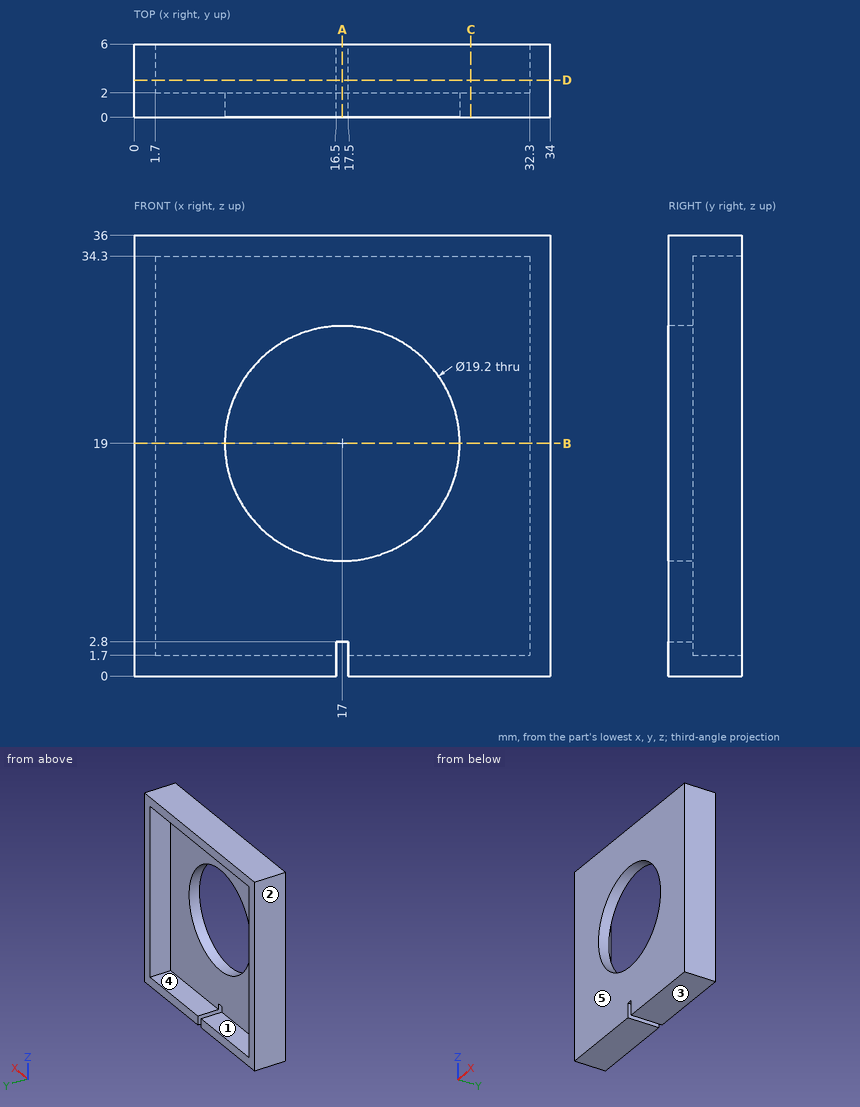
Design review of the part shown in the three views and the two pictorial views. Dimensions are in mm from the part's minimum x, y and z. A direction names the side the tool comes from. Coordinates: 2 decimals unless noted, no trailing zeros. Loops run counter-clockwise (first coordinate to the right, second up) from the corner with the lowest first, then second, coordinate; pieces in that order, holes last. Notation, with made-up numbers: M 21,-8 L 64,-8 A14 ccw 64,4 Z; hole C -30,-10 d5. An arc over 180 degrees is marked long. Put each result on its own line as item: value. Start each with the question number.
Q1. Add section C-C (x = 27.5). Write out the cut boundary in (y, z), and give its area (3 significant figures).
Q2. For the marked faces 4 and 5, list the 3-axis set-ups (+Z, -Z, +X, -X, +Y, -Y) from which the entire face can be reached by the end or side of a thin tool; tool diameter is ignored.
Q3. Add section B-B (z = 19). Write out the cut boundary in (x, y).
Q4. The part is to be moulded in two halves that separate along X. For the marked faces 1, 2 and 3, say which applies: +X half, -X half, draft (parallel to the pull), parting line (faces both ways), or undercut.
Q5. Add section D-D (y = 3.05). Write out the cut boundary in (x, z).
Q6. Clearance check with a flat-ended pin moving along its axis: pin 1 (3 mm diameter, centred on x = 18.5, z = 10, fed in from +Y). State where the tip first meets the part, or that it passes through.
Q7. Add section A-A (x = 17). Write out the cut boundary in (y, z).
Q8. Wall thickness on line 1 (X direction, y = 0.8, z = 19); line 2 (X direction, y = 5.25, z = 6); line 3 (Z direction, x = 4.5, y = 2.8): over which ranges is each line inside the solid? List them lowest first.
Answers:
1. outline: M 0,0 L 6,0 L 6,1.7 L 2,1.7 L 2,34.3 L 6,34.3 L 6,36 L 0,36 Z
1. area: 85.6 mm^2
2. face 4: +Y
2. face 5: +Z, -Z, +X, -X, -Y
3. outline: M 0,0 L 7.4,0 L 7.4,2 L 1.7,2 L 1.7,6 L 0,6 Z; M 26.6,0 L 34,0 L 34,6 L 32.3,6 L 32.3,2 L 26.6,2 Z
4. face 1: undercut
4. face 2: -X half
4. face 3: draft
5. outline: M 0,0 L 16.5,0 L 16.5,1.7 L 1.7,1.7 L 1.7,34.3 L 32.3,34.3 L 32.3,1.7 L 17.5,1.7 L 17.5,0 L 34,0 L 34,36 L 0,36 Z
6. pin 1: stops at y = 2
7. outline: M 0,2.8 L 2,2.8 L 2,9.4 L 0,9.4 Z; M 0,28.6 L 2,28.6 L 2,34.3 L 6,34.3 L 6,36 L 0,36 Z
8. line 1: x = 0 to 7.4, 26.6 to 34
8. line 2: x = 0 to 1.7, 32.3 to 34
8. line 3: z = 0 to 1.7, 34.3 to 36
